```python
from build123d import *

# Parameters (mm, degrees)
SKETCH2_R           = 2.2225
BOSS_EXTRUDE1_DEPTH = 6.35
SKETCH3_W           = 7.62
SKETCH3_H           = 40.64
SKETCH3_W_2         = 40.64
SKETCH3_H_2         = 7.62
BOSS_EXTRUDE2_DEPTH = 77.47
BOSS_EXTRUDE5_DEPTH = 40.64
BOSS_EXTRUDE6_DEPTH = 40.64
SKETCH8_R           = 3.937
CUT_EXTRUDE1_DEPTH  = 2.54


with BuildPart() as part:
    # Sketch2 → Boss-Extrude1 (new body)
    with BuildSketch(Plane(origin=(0, 0, 0), x_dir=(0, 0, -1), z_dir=(1, 0, 0))):
        with BuildLine():
            Line((-20.32, 98.425), (-20.32, 45.72))
            ThreePointArc((-20.32, 45.72), (-27.759487758, 27.759487758), (-45.72, 20.32))
            Line((-45.72, 20.32), (-90.805, 20.32))
            Line((-90.805, 20.32), (-90.805, -20.32))
            Line((-90.805, -20.32), (-45.72, -20.32))
            ThreePointArc((-45.72, -20.32), (-27.759487758, -27.759487758), (-20.32, -45.72))
            Line((-20.32, -45.72), (-20.32, -98.425))
            Line((-20.32, -98.425), (20.32, -98.425))
            Line((20.32, -98.425), (20.32, -45.72))
            ThreePointArc((20.32, -45.72), (27.759487758, -27.759487758), (45.72, -20.32))
            Line((45.72, -20.32), (90.805, -20.32))
            Line((90.805, -20.32), (90.805, 20.32))
            Line((90.805, 20.32), (45.72, 20.32))
            ThreePointArc((45.72, 20.32), (27.759487758, 27.759487758), (20.32, 45.72))
            Line((20.32, 45.72), (20.32, 98.425))
            Line((20.32, 98.425), (-20.32, 98.425))
        make_face()
        with Locations((54.765086962, 0)):
            Circle(SKETCH2_R, mode=Mode.SUBTRACT)
        with Locations((-54.765086962, 0)):
            Circle(SKETCH2_R, mode=Mode.SUBTRACT)
    extrude(amount=BOSS_EXTRUDE1_DEPTH)

    # Sketch3 → Boss-Extrude2 (add)
    with BuildSketch(Plane.ZY):
        with Locations((-86.995, 0)):
            Rectangle(SKETCH3_W, SKETCH3_H)
        with Locations((0, 94.615)):
            Rectangle(SKETCH3_W_2, SKETCH3_H_2)
        with Locations((86.995, 0)):
            Rectangle(SKETCH3_W, SKETCH3_H)
        with Locations((0, -94.615)):
            Rectangle(SKETCH3_W_2, SKETCH3_H_2)
    extrude(amount=BOSS_EXTRUDE2_DEPTH)

    # Sketch6 → Boss-Extrude5 (add)
    with BuildSketch(Plane(origin=(0, -20.32, 0), x_dir=(-1, 0, 0), z_dir=(0, -1, 0))):
        Polygon((77.47, 90.805), (90.273301898, 90.805), (77.47, 78.001698102), align=None)
        Polygon((90.273301898, -90.805), (77.47, -78.001698102), (77.47, -90.805), align=None)
    extrude(amount=-BOSS_EXTRUDE5_DEPTH)

    # Sketch7 → Boss-Extrude6 (add)
    with BuildSketch(Plane(origin=(0, 0, -20.32), x_dir=(-1, 0, 0), z_dir=(0, 0, -1))):
        Polygon((77.47, -98.425), (90.148305193, -98.425), (77.47, -85.746694807), align=None)
        Polygon((90.148305193, 98.425), (77.47, 85.746694807), (77.47, 98.425), align=None)
    extrude(amount=-BOSS_EXTRUDE6_DEPTH)

    # Sketch8 → Cut-Extrude1 (cut)
    with BuildSketch(Plane.ZY):
        with Locations((54.765086962, 0)):
            Circle(SKETCH8_R)
        with Locations(Location((-54.765086962, 0, 0), (0, 0, 180))):
            Circle(SKETCH8_R)
    extrude(amount=-CUT_EXTRUDE1_DEPTH, mode=Mode.SUBTRACT)


solid = part.part
```
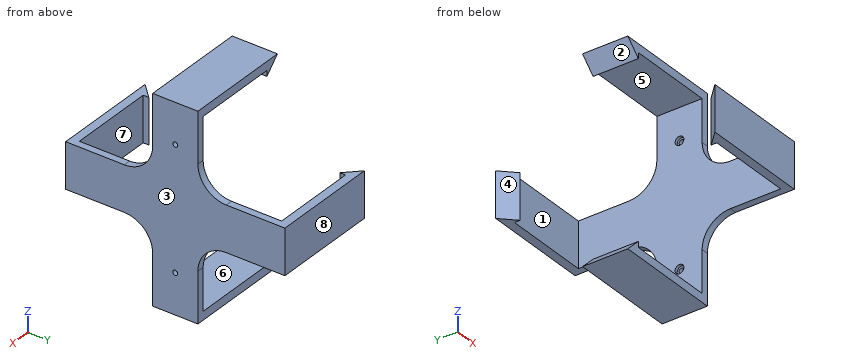
Geometry check sheet. Reference: the model listing, model coordinates, mm. Face numbers are marked on the shaded views. A direction names the side the tool comes from. Give positions to 0.01 mm unless a question says otherwise; leave off trailing zeros. Order: outer loops, then holes, each group sorted by start corner. A loop starts at its lowest first (then second) coordinate and runs counter-clockwise, first axis right, second up.
1. Section check A-A, the plane x = -24. Enter the section's corners in (y, z) (3 decimals), and give its area (3 significant figures).
2. Thickness scan on L1, parallel to Z at x = 3, y = 0 (3 decimals); L2, parallel to Z at x = -62, y = -11 (3 decimals); L3, parallel to Y at x = -72.5, z = -4 (3 decimals). Record the ranges inside material, lowest first.
3. Section check C-C, the plane x = -82. Enter the section's corners in (y, z) (3 decimals).
4. Access from +Z, -Z, +X, -X, +Y, -Y to the whole of each face (thin tool, end or side, straight path). Record for the marked faces 1, 2, 3, 4 and 5.
5. Gauge pin test, flat end, axial feed: pin 1 Ø2.5 at (y, z) = (0.5, 53) entering from -X. Record the tip position at first contact, or that the pin passes through.
6. Section check D-D, the plane z = -26.5. Enter the section's corners in (x, y), and give its area (3 significant figures).
7. Release check for a two-part mould opening along Y. For the marked faces 6, 7 and 8 record: pulls with the +Y half, pulls with the -Y half, needs draft (parallel to the pull), parting line crosses it, or undercut.
8. Section check B-B, the plane z = 74. Enter the section's corners in (x, y).
Values follow:
1. outline: (-98.425, -20.32) - (-90.805, -20.32) - (-90.805, 20.32) - (-98.425, 20.32) - close; (-20.32, -90.805) - (20.32, -90.805) - (20.32, -83.185) - (-20.32, -83.185) - close; (-20.32, 83.185) - (20.32, 83.185) - (20.32, 90.805) - (-20.32, 90.805) - close; (90.805, -20.32) - (98.425, -20.32) - (98.425, 20.32) - (90.805, 20.32) - close
1. area: 1,240 mm2
2. L1: z = -90.805 to -56.988, -52.543 to 52.543, 56.988 to 90.805
2. L2: z = -90.805 to -83.185, 83.185 to 90.805
2. L3: y = -98.425 to -90.805, 90.805 to 98.425
3. outline: (-98.425, -20.32) - (-90.277, -20.32) - (-90.277, 20.32) - (-98.425, 20.32) - close; (-20.32, -90.805) - (20.32, -90.805) - (20.32, -82.532) - (-20.32, -82.532) - close; (-20.32, 82.532) - (20.32, 82.532) - (20.32, 90.805) - (-20.32, 90.805) - close; (90.277, -20.32) - (98.425, -20.32) - (98.425, 20.32) - (90.277, 20.32) - close
4. face 1: +Z, -Z
4. face 2: -X, +Y, -Y
4. face 3: +Z, -Z, +X, +Y, -Y
4. face 4: +Z, -Z, -X
4. face 5: +Y, -Y
5. pin 1: stops at x = 2.54
6. outline: (0, -29.11) - (6.35, -29.11) - (6.35, 29.11) - (0, 29.11) - close
6. area: 370 mm2
7. face 6: needs draft
7. face 7: undercut
7. face 8: pulls with the +Y half
8. outline: (0, -20.32) - (6.35, -20.32) - (6.35, 20.32) - (0, 20.32) - close
